from build123d import *

# Parameters (mm, degrees)
F1_DEPTH = 25.4
F3_DEPTH = 12.7
F5_DEPTH = 25.401


with BuildPart() as f1:
    # F0 (on Front) → F1 (new body)
    with BuildSketch(Plane.XZ):
        Polygon((29.228445, 34.023839), (-28.236794, 34.024957), (-28.236794, -10.425043), (28.913206, -10.425043), align=None)
    extrude(amount=F1_DEPTH)

    # F2 (on face) → F3 (cut)
    with BuildSketch(Plane.XZ.offset(25.4)):
        Polygon((29.228445, 34.023839), (-9.186794, 34.024587), (16.213206, -10.425043), (28.913206, -10.425043), align=None)
    extrude(amount=-F3_DEPTH, mode=Mode.SUBTRACT)

    # F4 (on face) → F5 (cut, through all)
    with BuildSketch(Plane.XZ.offset(25.4)):
        with BuildLine():
            Line((-2.836794, 14.974957), (-15.536794, 14.974957))
            ThreePointArc((-15.536794, 14.974957), (-11.81705, 5.994701), (-2.836794, 2.274957))
            Line((-2.836794, 2.274957), (-2.836794, 14.974957))
        make_face()
        with BuildLine():
            Line((6.572767, 6.445586), (-5.408103, 27.411933))
            ThreePointArc((-5.408103, 27.411933), (-12.684271, 22.994757), (-15.536794, 14.974957))
            Line((-15.536794, 14.974957), (-2.836794, 14.974957))
            Line((-2.836794, 14.974957), (-2.836794, 2.274957))
            ThreePointArc((-2.836794, 2.274957), (2.309418, 3.364337), (6.572767, 6.445586))
        make_face()
        with BuildLine():
            ThreePointArc((6.572767, 6.445586), (9.012076, 10.40393), (9.863206, 14.974957))
            ThreePointArc((9.863206, 14.974957), (5.183006, 24.822435), (-5.408103, 27.411933))
            Line((-5.408103, 27.411933), (6.572767, 6.445586))
        make_face()
    extrude(amount=-F5_DEPTH, mode=Mode.SUBTRACT)


solid = f1.part
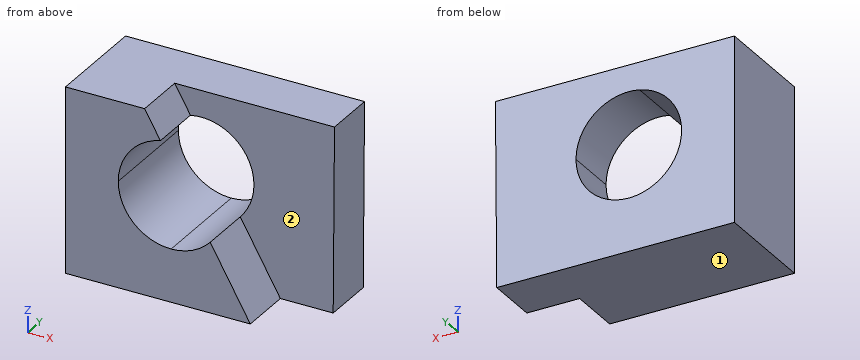
Geometry: final body of the model. Coordinates: model frame, mm. Face numbers are marked on the shaded views. A direction names the side the tool comes from. Round coordinates to 2 decimals unless told otherwise and drop trailing zeros. Order: outer loops, then holes, each group sorted by start corner. A loop starts at its lowest first (then second) coordinate and runs counter-clockwise, first axis right, second up. Notation, with made-up numbers: (26, 86) - (36, 86) arc R19 cw to (36, 93) - close; hole circle Ø3 at (-16, 67.25). An arc over 180 degrees is marked (long way). Write each question's results on one line, items separated by ' | '.
Item 1: Section C-C, the plane y = -22.25. Return the cut outline in (x, z), and give its area (3 significant figures).
Completed:
outline: (-28.24, -10.43) - (16.21, -10.43) - (6.57, 6.45) arc R12.7 cw to (-2.84, 2.27) arc R12.7 cw to (-5.41, 27.41) - (-9.19, 34.02) - (-28.24, 34.02) - close | area: 1,060 mm^2
Item 2: Section B-B, the plane x = -1.5. Return the cut outline in (y, z).
Completed:
outline: (-25.4, -10.43) - (0, -10.43) - (0, 2.35) - (-25.4, 2.35) - close; (-12.7, 27.6) - (0, 27.6) - (0, 34.02) - (-12.7, 34.02) - close
Item 3: Section D-D, the plane z = 17.5. Return the cut outline in (x, y).
Completed:
outline: (-28.24, -25.4) - (-15.28, -25.4) - (-15.28, 0) - (-28.24, 0) - close; (9.61, -12.7) - (29.11, -12.7) - (29.11, 0) - (9.61, 0) - close
Item 4: First-contact query: pin 1 Ø19 at (x, z) = (14, 20.5) entering from -Y; pin 2 Ø10 at (x, z) = (9, 8.5) entering from -Y; pin 3 Ø8 at (x, y) = (17, -18.5) entering from +Z; pin 4 Ø2 at (x, y) = (12, -18) entering from +Z. Flat tips, straight axial feed; report the tip coordinate or a pass-through.
Completed:
pin 1: y = -12.7 | pin 2: y = -25.4 | pin 3: z = -4.8 | pin 4: z = -1.3
Item 5: Material intervals for line 1 along Y through (x, z) = (10, 15.5); line 2 along X through (y, z) = (-10, 17); line 3 along X through (y, z) = (-2.5, 5), sorted ascending. Write a range as [from, to].
Completed:
line 1: [-12.7, 0] | line 2: [-28.24, -15.37], [9.7, 29.11] | line 3: [-28.24, -10.7], [5.02, 29.02]
Item 6: Reachability of the marked faces 1 and 2 from +Z, -Z, +X, -X, +Y, -Y: full face, straight path, thin tool, end or side. Return the list, or none.
Completed:
face 1: -Z, +X, -X, +Y, -Y | face 2: +Z, +X, -Y
Item 7: Section A-A, the plane y = -8.75. Return the cut outline in (x, z), and give its area (3 significant figures).
Completed:
outline: (-28.24, -10.43) - (28.91, -10.43) - (29.23, 34.02) - (-28.24, 34.02) - close; hole (-5.41, 27.41) arc R12.7 ccw to (-2.84, 2.27) arc R12.7 ccw to (6.57, 6.45) arc R12.7 ccw to (9.86, 14.97) arc R12.7 ccw to start | area: 2,040 mm^2
